Part model, mm, in its own coordinate system. A direction names the side the tool comes from. Round coordinates to 2 decimals unless told otherwise and drop trailing zeros. Loops run counter-clockwise (first coordinate to the right, second up) from the corner with the lowest first, then second, coordinate; pieces in that order, holes last.
from build123d import *

# Parameters (mm, degrees)
ESQUISSE1_W             = 16
ESQUISSE1_H             = 16
EXTRUSION1_DEPTH        = 12.5
CONG_1_R                = 1
ESQUISSE2_R             = 5
EXTRUSION2_DEPTH        = 9
CHANFREIN1_SIZE         = 1
ESQUISSE3_R             = 3
EXTRUSION3_DEPTH        = 13
ESQUISSE4_W             = 6.995230525
ESQUISSE4_H             = 1
ENL_V_MAT_EXTRU_1_DEPTH = 2
ENL_V_MAT_EXTRU_2_DEPTH = 1
ENL_V_START             = -1
ENL_V_MAT_EXTRU_3_DEPTH = 1


with BuildPart() as part:
    # Esquisse1 → Extrusion1 (new body)
    with BuildSketch(Plane.XY):
        with Locations((8, 8)):
            Rectangle(ESQUISSE1_W, ESQUISSE1_H)
    extrude(amount=EXTRUSION1_DEPTH)

    # Congé1
    cong_1_edges = [part.edges().sort_by_distance(p)[0] for p in [
        (0, 16, 6.25),
        (16, 16, 6.25),
        (16, 0, 6.25),
        (0, 0, 6.25),
    ]]
    fillet(cong_1_edges, radius=CONG_1_R)

    # Esquisse2 → Extrusion2 (add)
    with BuildSketch(Plane.XY.offset(12.5)):
        with Locations(Location((8, 8, 0), (0, 0, 180))):
            Circle(ESQUISSE2_R)
    extrude(amount=EXTRUSION2_DEPTH)

    # Chanfrein1
    chanfrein1_edges = [part.edges().sort_by_distance(p)[0] for p in [
        (13, 8, 21.5),
    ]]
    chamfer(chanfrein1_edges, length=CHANFREIN1_SIZE)

    # Esquisse3 → Extrusion3 (add)
    with BuildSketch(Plane.XY.offset(21.5)):
        with Locations(Location((8, 8, 0), (0, 0, 180))):
            Circle(ESQUISSE3_R)
    extrude(amount=EXTRUSION3_DEPTH)

    # Esquisse4 → Enlèv. mat.-Extru.1 (cut)
    with BuildSketch(Plane.XY.offset(34.5)):
        with Locations((8.099931865, 8)):
            Rectangle(ESQUISSE4_W, ESQUISSE4_H)
    extrude(amount=-ENL_V_MAT_EXTRU_1_DEPTH, mode=Mode.SUBTRACT)

    # Esquisse5 → Enlèv. mat.-Extru.2 (cut)
    with BuildSketch(Plane.XY.offset(12.5)):
        with BuildLine():
            Line((13, 17.678512004), (13, 14))
            ThreePointArc((13, 14), (13.292893219, 13.292893219), (14, 13))
            Line((14, 13), (16.806932946, 13))
            Line((16.806932946, 13), (16.806932946, 17.678512004))
            Line((16.806932946, 17.678512004), (13, 17.678512004))
        make_face()
        with BuildLine():
            Line((-0.806932946, 17.678512004), (3, 17.678512004))
            Line((3, 17.678512004), (3, 14))
            ThreePointArc((3, 14), (2.707106781, 13.292893219), (2, 13))
            Line((2, 13), (-0.806932946, 13))
            Line((-0.806932946, 13), (-0.806932946, 17.678512004))
        make_face()
        with BuildLine():
            Line((16.806932946, -1.678512004), (13, -1.678512004))
            Line((13, -1.678512004), (13, 2))
            ThreePointArc((13, 2), (13.292893219, 2.707106781), (14, 3))
            Line((14, 3), (16.806932946, 3))
            Line((16.806932946, 3), (16.806932946, -1.678512004))
        make_face()
        with BuildLine():
            Line((3, -1.678512004), (3, 2))
            ThreePointArc((3, 2), (2.707106781, 2.707106781), (2, 3))
            Line((2, 3), (-0.806932946, 3))
            Line((-0.806932946, 3), (-0.806932946, -1.678512004))
            Line((-0.806932946, -1.678512004), (3, -1.678512004))
        make_face()
    extrude(amount=-ENL_V_MAT_EXTRU_2_DEPTH, mode=Mode.SUBTRACT)

    # Esquisse6 → Enlèv. mat.-Extru.3 (cut)
    with BuildSketch(Plane(origin=(0, 0, 0), x_dir=(-1, 0, 0), z_dir=(0, 0, -1)).offset(ENL_V_START)):
        with BuildLine():
            Line((0, 13), (0, 15))
            ThreePointArc((0, 15), (-0.292893219, 15.707106781), (-1, 16))
            Line((-1, 16), (-3, 16))
            Line((-3, 16), (-3, 14))
            ThreePointArc((-3, 14), (-2.707106781, 13.292893219), (-2, 13))
            Line((-2, 13), (0, 13))
        make_face()
        with BuildLine():
            Line((-13, 16), (-15, 16))
            ThreePointArc((-15, 16), (-15.707106781, 15.707106781), (-16, 15))
            Line((-16, 15), (-16, 13))
            Line((-16, 13), (-14, 13))
            ThreePointArc((-14, 13), (-13.292893219, 13.292893219), (-13, 14))
            Line((-13, 14), (-13, 16))
        make_face()
        with BuildLine():
            Line((-3, 0), (-1, 0))
            ThreePointArc((-1, 0), (-0.292893219, 0.292893219), (0, 1))
            Line((0, 1), (0, 3))
            Line((0, 3), (-2, 3))
            ThreePointArc((-2, 3), (-2.707106781, 2.707106781), (-3, 2))
            Line((-3, 2), (-3, 0))
        make_face()
        with BuildLine():
            Line((-15, 0), (-13, 0))
            Line((-13, 0), (-13, 2))
            ThreePointArc((-13, 2), (-13.292893219, 2.707106781), (-14, 3))
            Line((-14, 3), (-16, 3))
            Line((-16, 3), (-16, 1))
            ThreePointArc((-16, 1), (-15.707106781, 0.292893219), (-15, 0))
        make_face()
    extrude(amount=ENL_V_MAT_EXTRU_3_DEPTH, mode=Mode.SUBTRACT)


solid = part.part
1) Tool access for faces 5 (the face through (3, 1, 0.5)), 6 (the face through (1, 13, 0.5)), 7 (the face through (4, 12, 12.5)): list every direction of +Z, -Z, +X, -X, +Y, -Y with a clear straight run to the whole face (end or side of a thin tool).
Values:
face 5: -Z, -X, -Y
face 6: -Z, -X, +Y
face 7: +Z
2) Slice it at A-A, the plane y = 14.5. Give the cut face in (x, z), then the cut area to 3 significant figures.
Values:
outline: (0, 1) - (3, 1) - (3, 0) - (13, 0) - (13, 1) - (16, 1) - (16, 11.5) - (13, 11.5) - (13, 12.5) - (3, 12.5) - (3, 11.5) - (0, 11.5) - close
area: 188 mm2
3) Slice it at B-B, the plane x = 8. Give the cut face in (y, z), then the cut area to 3 significant figures.
Values:
outline: (0, 0) - (16, 0) - (16, 12.5) - (13, 12.5) - (13, 20.5) - (12, 21.5) - (11, 21.5) - (11, 34.5) - (8.5, 34.5) - (8.5, 32.5) - (7.5, 32.5) - (7.5, 34.5) - (5, 34.5) - (5, 21.5) - (4, 21.5) - (3, 20.5) - (3, 12.5) - (0, 12.5) - close
area: 365 mm2
4) Slice it at C-C, the plane z = 23. Give the cut face in (x, y).
Values:
outline: circle Ø6 at (8, 8)
5) Mould opens along Y. For faces 1 (the face through (13, 15, 0.5)), 2 (the face through (8, 8.5, 34)), 3 (the face through (2.715, 13.301, 12.007)), 4 (the face through (15, 3, 0.5)) say: released by +Y, released by -Y, zero draft, split by the parting line, or undercut.
Values:
face 1: zero draft
face 2: undercut
face 3: released by +Y
face 4: released by -Y
6) Slice it at D-D, the plane y = 8. Give the cut face in (x, z).
Values:
outline: (0, 0) - (16, 0) - (16, 12.5) - (13, 12.5) - (13, 20.5) - (12, 21.5) - (11, 21.5) - (11, 32.5) - (5, 32.5) - (5, 21.5) - (4, 21.5) - (3, 20.5) - (3, 12.5) - (0, 12.5) - close
7) Wall check: line 1 along Z through (x, y) = (7.25, 14.5); line 2 along Z through (x, y) = (11, 10); line 3 along Y through (x, z) = (7.5, 25). Give the ranges that are in metal, low to high.
Values:
line 1: z = 0 to 12.5
line 2: z = 0 to 21.5
line 3: y = 5.04 to 10.96
8) Drop flat-ended pins along their axis: pin 1 Ø8 at (y, z) = (5, 17.5) entering from +X; pin 2 Ø3.5 at (x, y) = (14, 15) entering from +Z; pin 3 Ø3.5 at (x, y) = (1, 1) entering from +Z; pin 4 Ø1.1 at (y, z) = (15, 0.5) entering from +X. Give the stop position or say it passes through.
Values:
pin 1: stops at x = 13
pin 2: stops at z = 12.5
pin 3: stops at z = 11.5
pin 4: stops at x = 16
